```python
from build123d import *

# Parameters (mm, degrees)
SKETCH1_W           = 19.1
SKETCH1_H           = 19.1
BOSS_EXTRUDE1_DEPTH = 6.4
SKETCH2_R           = 4.75
BOSS_EXTRUDE2_DEPTH = 76.2
SKETCH3_OUTSIDE_W   = 51.28
SKETCH3_OUTSIDE_H   = 51.28
SKETCH3_OUTSIDE_R   = 9.55
CUT_EXTRUDE2_DEPTH  = 6.4
CUT_EXTRUDE2_DRAFT  = -45


with BuildPart() as part:
    # Sketch1 → Boss-Extrude1 (new body)
    with BuildSketch(Plane.XY):
        Rectangle(SKETCH1_W, SKETCH1_H)
    extrude(amount=-BOSS_EXTRUDE1_DEPTH)

    # Sketch2 → Boss-Extrude2 (add)
    with BuildSketch(Plane(origin=(0, 0, -6.4), x_dir=(-1, 0, 0), z_dir=(0, 0, -1))):
        with Locations(Location((0, 0, 0), (0, 0, 180))):
            Circle(SKETCH2_R)
    extrude(amount=BOSS_EXTRUDE2_DEPTH)


with BuildPart() as cut_extrude2_tool:
    # Sketch3 outside → Cut-Extrude2 (with draft: the straight prism first)
    with BuildSketch(Plane.XY):
        Rectangle(SKETCH3_OUTSIDE_W, SKETCH3_OUTSIDE_H)
        Circle(SKETCH3_OUTSIDE_R, mode=Mode.SUBTRACT)
    extrude(amount=-CUT_EXTRUDE2_DEPTH)
    # Cut-Extrude2: the draft: its side faces are tilted about the plane it starts from
    cut_extrude2_sides = [cut_extrude2_tool.faces().sort_by_distance(p)[0] for p in [
        (0, -25.64, -3.2),
        (25.64, 0, -3.2),
        (0, 25.64, -3.2),
        (-25.64, 0, -3.2),
        (-9.55, 0, -3.2),
    ]]
    draft(cut_extrude2_sides, Plane.XY, CUT_EXTRUDE2_DRAFT)


with BuildPart() as part_1:
    add(part.part)

    # Cut-Extrude2: cut by cut_extrude2_tool
    add(cut_extrude2_tool.part, mode=Mode.SUBTRACT)


solid = part_1.part
```
Read the model definition and answer for the solid it produces. Units are mm, in the model's axes. A direction names the side the tool comes from. Give positions to 0.01 mm unless a question says otherwise; leave off trailing zeros. Write each loop counter-clockwise with the first axis right and the second up, starting at its lowest first coordinate (ties: lowest second). Pieces come first, ordered by that corner, then holes. Notation, with made-up numbers: M 51,13.25 L 65,13.25 A34 cw 65,43.25 Z; hole C 58,-18.75 d1. An arc over 180 degrees is marked long. Put each result on its own line as item: value. Start each with the question number.
1. The part is cut by section A-A, the plane z = -15. Give the vertices of the cut face in (x, y).
2. Each of these flat-tipped pins is pushed along its axis until it touches: pin 1 Ø3 at (x, z) = (5, -71.5) entering from +Y; pin 2 Ø3 at (x, z) = (4.5, -10) entering from -Y; pin 3 Ø1.5 at (y, z) = (4.5, -25) entering from +X. Where does it stop, or does it pass through?
3. Consider line 1 along Z through (x, y) = (-2.25, 7.75); line 2 along X through (y, z) = (3.5, -20); line 3 along Y through (x, z) = (-2.5, -68). Determine where each line is inside the solid, lowest interval first.
4. Which of the six approach directions +Z, -Z, +X, -X, +Y, -Y give full straight-line access (tool end or side, diameter ignored) to faces 1 (the cylindrical face through (-1.03, 4.637, -43.967)), 2 (the conical face through (7.447, 7.392, -0.943))?
Final values:
1. outline: C 0,0 d9.5
2. pin 1: stops at y = 3.21
2. pin 2: stops at y = -3.68
2. pin 3: stops at x = 2.92
3. line 1: z = -6.4 to 0
3. line 2: x = -3.21 to 3.21
3. line 3: y = -4.04 to 4.04
4. face 1: -Z
4. face 2: +Z, +X, +Y
